Check sheet for the modelled part. Datum: model origin and axes. Units: mm. Coordinates: 2 decimals unless noted, no trailing zeros. Write each loop counter-clockwise with the first axis right and the second up, starting at its lowest first coordinate (ties: lowest second). Pieces come first, ordered by that corner, then holes. Notation, with made-up numbers: (-9, -31.75) -> (47, -31.75) arc R11 ccw to (47, -25.75) -> close; hole circle Ø11 at (75, -8.75). An arc over 180 degrees is marked (long way). Put each result on its own line as item: value.
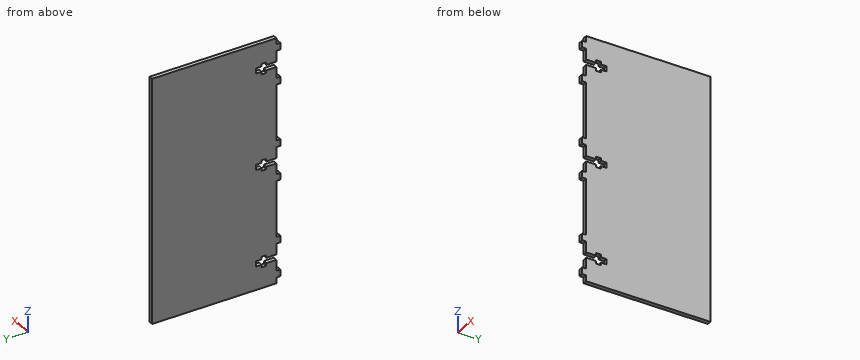
```python
from build123d import *

# Parameters (mm, degrees)
BOSS_EXTRUDE1_DEPTH = 3


with BuildPart() as part:
    # Sketch1 → Boss-Extrude1 (new, symmetric)
    with BuildSketch(Plane(origin=(0, 0, 0), x_dir=(0, 0, -1), z_dir=(1, 0, 0))):
        Polygon((185, 92.5), (-185, 92.5), (-185, -92.5), (-176, -92.5), (-176, -98.5), (-166, -98.5), (-166, -92.5), (-149.5, -92.5), (-149.5, -77.5), (-153.5, -77.5), (-153.5, -70.5), (-149.5, -70.5), (-149.5, -62.5), (-141.5, -62.5), (-141.5, -70.5), (-137.5, -70.5), (-137.5, -77.5), (-141.5, -77.5), (-141.5, -92.5), (-125, -92.5), (-125, -98.5), (-115, -98.5), (-115, -92.5), (-30.5, -92.5), (-30.5, -98.5), (-20.5, -98.5), (-20.5, -92.5), (-4, -92.5), (-4, -77.5), (-8, -77.5), (-8, -70.5), (-4, -70.5), (-4, -62.5), (4, -62.5), (4, -70.5), (8, -70.5), (8, -77.5), (4, -77.5), (4, -92.5), (20.5, -92.5), (20.5, -98.5), (30.5, -98.5), (30.5, -92.5), (115, -92.5), (115, -98.5), (125, -98.5), (125, -92.5), (141.5, -92.5), (141.5, -77.5), (137.5, -77.5), (137.5, -70.5), (141.5, -70.5), (141.5, -62.5), (149.5, -62.5), (149.5, -70.5), (153.5, -70.5), (153.5, -77.5), (149.5, -77.5), (149.5, -92.5), (166, -92.5), (166, -98.5), (176, -98.5), (176, -92.5), (185, -92.5), align=None)
    extrude(amount=BOSS_EXTRUDE1_DEPTH, both=True)


solid = part.part
```
Q1. Cross-section at B-B (z = -161.5). Record the cut outline in (x, y), plus the area to 3 significant figures.
Recorded:
outline: (-3, -92.5) -> (3, -92.5) -> (3, 92.5) -> (-3, 92.5) -> close
area: 1,110 mm2
Q2. Material ranges on line 1 along Y through (x, z) = (1.15, 128), recorded low to high.
Recorded:
line 1: y = -92.5 to 92.5
Q3. Depth check by flat-ended pin: P1, Ø1.2, axis at x = 1, z = 151.5, coming from the -Y side. Enter the tip coordinate at first touch or a pass-through.
Recorded:
P1: stops at y = -92.5
Q4. Cross-section at A-A (y = -74). Record the cut outline in (x, z).
Recorded:
outline: (-3, -185) -> (3, -185) -> (3, -153.5) -> (-3, -153.5) -> close; (-3, -137.5) -> (3, -137.5) -> (3, -8) -> (-3, -8) -> close; (-3, 8) -> (3, 8) -> (3, 137.5) -> (-3, 137.5) -> close; (-3, 153.5) -> (3, 153.5) -> (3, 185) -> (-3, 185) -> close
